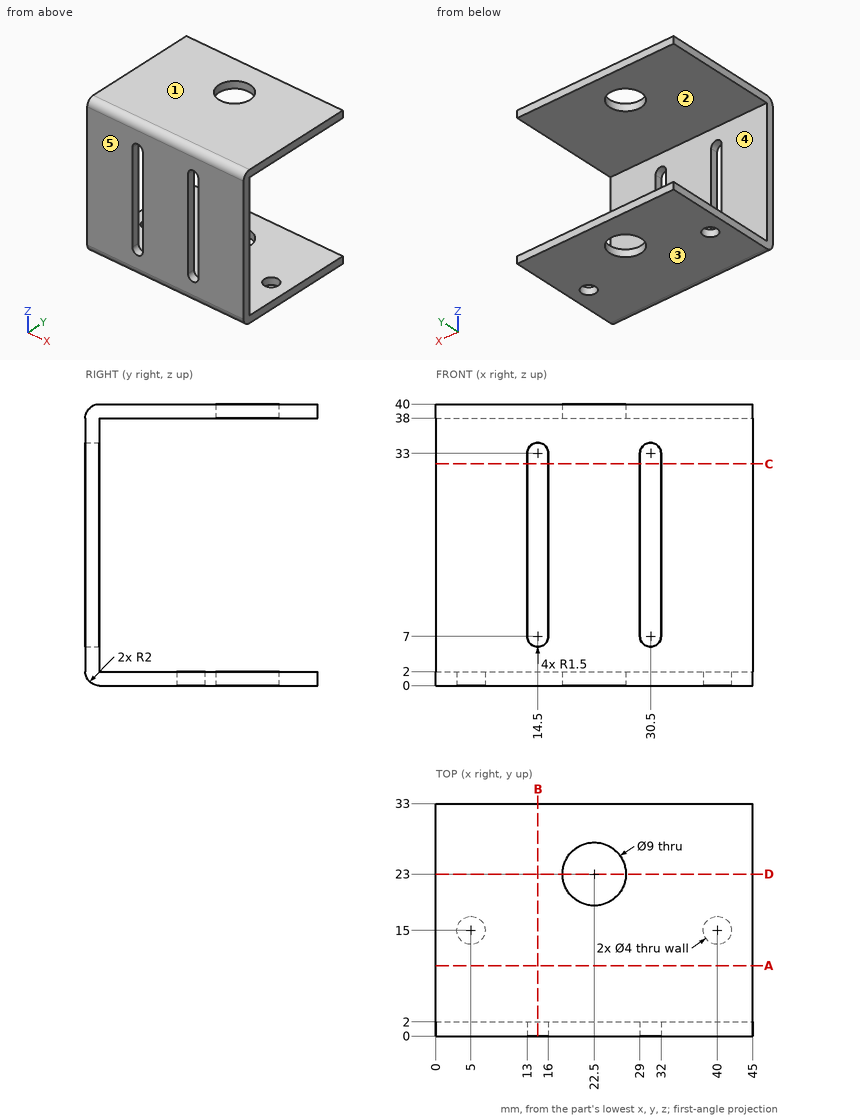
Geometry: see drawing. Coordinates: mm, zero at the bounding-box minimum. A direction names the side the tool comes from. Round coordinates to 2 decimals unless told otherwise and drop trailing zeros. Loops run counter-clockwise (first coordinate to the right, second up) from the corner with the lowest first, then second, coordinate; pieces in that order, holes last. Notation, with made-up numbers: (58.5, 44.5) -> (85.5, 44.5) arc R15 cw to (85.5, 70.5) -> close; hole circle Ø1 at (81.25, 33.5). An arc over 180 degrees is marked (long way). Write each question's results on one line, items separated by ' | '.
1. Mould query, pull axis Z, two halves, no side actions, for the marked faces 3, 4 and 5. Classes: +Z half, -Z half, draft (parallel to the pull), parting line (faces both ways), or undercut.
Geometry results:
face 3: -Z half | face 4: undercut | face 5: draft
2. Section D-D (y = 23). Return loops of the section in (x, z), and give its area (3 significant figures).
Geometry results:
outline: (0, 0) -> (18, 0) -> (18, 2) -> (0, 2) -> close; (0, 38) -> (18, 38) -> (18, 40) -> (0, 40) -> close; (27, 0) -> (45, 0) -> (45, 2) -> (27, 2) -> close; (27, 38) -> (45, 38) -> (45, 40) -> (27, 40) -> close | area: 144 mm2
3. Section B-B (x = 14.5). Return loops of the section in (y, z).
Geometry results:
outline: (0, 2) arc R2 ccw to (2, 0) -> (33, 0) -> (33, 2) -> (2, 2) -> (2, 5.5) -> (0, 5.5) -> close; (0, 34.5) -> (2, 34.5) -> (2, 38) -> (33, 38) -> (33, 40) -> (2, 40) arc R2 ccw to (0, 38) -> close
4. First-contact query: P1, Ø1, axis at y = 4, z = 24.5, coming from the -X side; P2, Ø2, axis at x = 21, z = 10, coming from the +Y side. Flat tips, straight axial feed; report the tip coordinate or a pass-through.
Geometry results:
P1: through | P2: y = 2
5. Section C-C (z = 31.5). Return loops of the section in (x, y).
Geometry results:
outline: (0, 0) -> (13, 0) -> (13, 2) -> (0, 2) -> close; (16, 0) -> (29, 0) -> (29, 2) -> (16, 2) -> close; (32, 0) -> (45, 0) -> (45, 2) -> (32, 2) -> close
6. Set-up query: the marked faces 1 and 2. Return all of +Z, -Z, +X, -X, +Y, -Y with unobstructed straight access to the full face (end or side cutting, diameter ignored); none if empty.
Geometry results:
face 1: +Z, +X, -X, +Y, -Y | face 2: +X, -X, +Y
7. Section A-A (y = 10). Return loops of the section in (x, z).
Geometry results:
outline: (0, 0) -> (45, 0) -> (45, 2) -> (0, 2) -> close; (0, 38) -> (45, 38) -> (45, 40) -> (0, 40) -> close
8. Ray query, line 1 (X direction, y = 15, z = 1); line 2 (Z direction, x = 10, y = 9); line 3 (Y direction, x = 16.5, z = 14). Return the intervals inside material, ascending. Write a range as from..to.
Geometry results:
line 1: 0..3, 7..38, 42..45 | line 2: 0..2, 38..40 | line 3: 0..2
